Geometry check sheet. Reference: the model listing, model coordinates, mm. A direction names the side the tool comes from. Round coordinates to 2 decimals unless told otherwise and drop trailing zeros. Write each loop counter-clockwise with the first axis right and the second up, starting at its lowest first coordinate (ties: lowest second). Pieces come first, ordered by that corner, then holes. Notation, with made-up numbers: M 33.5,-34 L 78.5,-34 A7 ccw 78.5,-27 Z; hole C 20,58 d11. An arc over 180 degrees is marked long. One line per item, written item: value. Start each with the question number.
1. Release check for a two-part mould opening along X. For faces 6 (the flat face through (-30, 3, 25.921)), 7 (the cylindrical face through (-44.33, 14.18, 34.82)), 8 (the cylindrical face through (-19.545, 8.715, 19.022)) record: pulls with the +X half, pulls with the -X half, needs draft (parallel to the pull), parting line crosses it, or undercut.
2. Scan lines: probe 1 along Z at (x, y) = (-20, 6.5); probe 2 along Z at (x, y) = (-38.5, 21.5); probe 3 along Y at (x, z) = (-17.5, 24). Record each from-to range of solid material in increasing order. Write a range as [from, to].
3. Section check D-D (y = 20.75). Record the boundary of the cut face in (x, z).
4. Section check C-C (x = -20). Record the boundary of the cut face in (y, z), and give its area (3 significant figures).
5. Access from +Z, -Z, +X, -X, +Y, -Y to the whole of each face (thin tool, end or side, straight path). Record for faces 1 (the flat face through (-14.615, 9, 32)), 2 (the flat face through (-29, 16, 31.699)), 3 (the flat face through (-40, 9, 22)), 4 (the flat face through (-24.615, 5, 22)), 5 (the cylindrical face through (-34.9, 0.3, 23.4)).
6. Section check A-A (y = 12). Record the boundary of the cut face in (x, z), and give its area (3 significant figures).
7. Section check B-B (z = 25.25). Record the boundary of the cut face in (x, y), and give its area (3 significant figures).
8. Depth check by flat-ended pin: P1, Ø2.5, axis at x = -34.61, y = 12, coming from the +Z side; P2, Ø3.5, axis at x = -24.61, y = 12, coming from the +Z side; P3, Ø2, axis at x = -30, y = 3, coming from the -Z side; P4, Ø1.2, axis at x = -19, z = 21.5, coming from the +Y side. Enter the tip coordinate at first touch or a pass-through.
from build123d import *

# Parameters (mm, degrees)
BOSS_EXTRUDE1_DEPTH = 5
SKETCH1_3_W         = 10
SKETCH1_3_H         = 5
BOSS_EXTRUDE2_DEPTH = 9
BOSS_EXTRUDE3_DEPTH = 22
SKETCH4_R           = 1.6
CUT_EXTRUDE1_DEPTH  = 3.424711692
FILLET1_R           = 1
FILLET2_R           = 1


with BuildPart() as part:
    # Sketch1 → Boss-Extrude1 (new body)
    with BuildSketch(Plane(origin=(0, 0, 0), x_dir=(1, 0, 0), z_dir=(0, 1, 0))):
        Polygon((-44.61462686, -35.123247006), (-14.61462686, -35.123247006), (-14.61462686, -18.720861087), (-24.61462686, -18.720861087), (-24.61462686, -25.920861087), (-34.61462686, -25.920861087), (-34.61462686, -18.720861087), (-44.61462686, -18.720861087), align=None)
    extrude(amount=BOSS_EXTRUDE1_DEPTH)

    # Sketch1<3> → Boss-Extrude2 (add)
    with BuildSketch(Plane(origin=(0, 0, 0), x_dir=(1, 0, 0), z_dir=(0, 1, 0))):
        with Locations((-39.61462686, -21.220861087)):
            Rectangle(SKETCH1_3_W, SKETCH1_3_H)
        with Locations((-19.61462686, -21.220861087)):
            Rectangle(SKETCH1_3_W, SKETCH1_3_H)
    extrude(amount=BOSS_EXTRUDE2_DEPTH)

    # Sketch3 → Boss-Extrude3 (add)
    with BuildSketch(Plane(origin=(0, 5, 0), x_dir=(1, 0, 0), z_dir=(0, 1, 0))):
        Polygon((-34.61462686, -31.698535314), (-44.61462686, -31.698535314), (-44.61462686, -35.123247006), (-14.61462686, -35.123247006), (-14.61462686, -31.698535314), align=None)
    extrude(amount=BOSS_EXTRUDE3_DEPTH)

    # Sketch4 → Cut-Extrude1 (cut)
    with BuildSketch(Plane(origin=(0, 0, 31.698535314), x_dir=(-1, 0, 0), z_dir=(0, 0, -1))):
        with Locations((34.61462686, 12)):
            Circle(SKETCH4_R)
        with Locations((24.61462686, 12)):
            Circle(SKETCH4_R)
    extrude(amount=-CUT_EXTRUDE1_DEPTH, mode=Mode.SUBTRACT)

    # Fillet1
    fillet1_edges = [part.edges().sort_by_distance(p)[0] for p in [
        (-33.01462686, 12, 31.698535314),
        (-33.01462686, 12, 35.123247006),
        (-23.01462686, 12, 31.698535314),
        (-23.01462686, 12, 35.123247006),
    ]]
    fillet(fillet1_edges, radius=FILLET1_R)

    # Fillet2
    fillet2_edges = [part.edges().sort_by_distance(p)[0] for p in [
        (-39.61462686, 0, 18.720861087),
        (-34.61462686, 0, 22.320861087),
        (-29.61462686, 0, 25.920861087),
        (-24.61462686, 0, 22.320861087),
        (-19.61462686, 0, 18.720861087),
        (-14.61462686, 0, 26.922054046),
        (-14.61462686, 13.5, 35.123247006),
        (-44.61462686, 13.5, 35.123247006),
        (-44.61462686, 4.5, 18.720861087),
        (-34.61462686, 4.5, 18.720861087),
        (-24.61462686, 4.5, 18.720861087),
        (-14.61462686, 4.5, 18.720861087),
        (-39.61462686, 9, 18.720861087),
        (-19.61462686, 9, 18.720861087),
        (-29.61462686, 27, 35.123247006),
        (-29.61462686, 0, 35.123247006),
        (-44.61462686, 0, 26.922054046),
    ]]
    fillet(fillet2_edges, radius=FILLET2_R)


solid = part.part
Result sheet:
1. face 6: undercut
1. face 7: pulls with the -X half
1. face 8: needs draft
2. probe 1: z = [18.72, 23.72], [31.7, 35.12]
2. probe 2: z = [31.7, 35.12]
2. probe 3: y = [0, 5]
3. outline: M -44.61,31.7 L -14.61,31.7 L -14.61,34.12 A1 ccw -15.61,35.12 L -43.61,35.12 A1 ccw -44.61,34.12 Z
4. outline: M 0,19.72 A1 ccw 1,18.72 L 8,18.72 A1 ccw 9,19.72 L 9,23.72 L 5,23.72 L 5,31.7 L 27,31.7 L 27,34.12 A1 ccw 26,35.12 L 1,35.12 A1 ccw 0,34.12 Z
4. area: 176 mm2
5. face 1: +Z, -Z, +X, +Y, -Y
5. face 2: +X, -X, +Y
5. face 3: -Z, +X, -X, +Y
5. face 4: -Z, +Y, -Y
5. face 5: -Z, -Y
6. outline: M -44.61,31.7 L -37.21,31.7 A1 ccw -36.21,32.7 L -36.21,34.12 A1 ccw -37.21,35.12 L -43.61,35.12 A1 ccw -44.61,34.12 Z; M -33.01,32.7 A1 ccw -32.01,31.7 L -27.21,31.7 A1 ccw -26.21,32.7 L -26.21,34.12 A1 ccw -27.21,35.12 L -32.01,35.12 A1 ccw -33.01,34.12 Z; M -23.01,32.7 A1 ccw -22.01,31.7 L -14.61,31.7 L -14.61,34.12 A1 ccw -15.61,35.12 L -22.01,35.12 A1 ccw -23.01,34.12 Z
6. area: 78.7 mm2
7. outline: M -44.61,1 A1 ccw -43.61,0 L -35.61,0 A1 ccw -34.61,1 L -34.61,5 L -44.61,5 Z; M -24.61,1 A1 ccw -23.61,0 L -15.61,0 A1 ccw -14.61,1 L -14.61,5 L -24.61,5 Z
7. area: 99.1 mm2
8. P1: passes through
8. P2: stops at z = 34.66
8. P3: stops at z = 25.92
8. P4: stops at y = 9
